Design review of the part built by this model. Coordinates are the model's own, in mm. Face numbers are marked on the shaded views. A direction names the side the tool comes from. Give positions to 0.01 mm unless a question says otherwise; leave off trailing zeros. Order: outer loops, then holes, each group sorted by start corner. A loop starts at its lowest first (then second) coordinate and runs counter-clockwise, first axis right, second up. Notation, with made-up numbers: (54, 74.5) -> (103, 74.5) arc R23 ccw to (103, 105.5) -> close; hole circle Ø9 at (-5, 12.25). An arc over 180 degrees is marked (long way). Return JSON: item names as keys, results as strings.
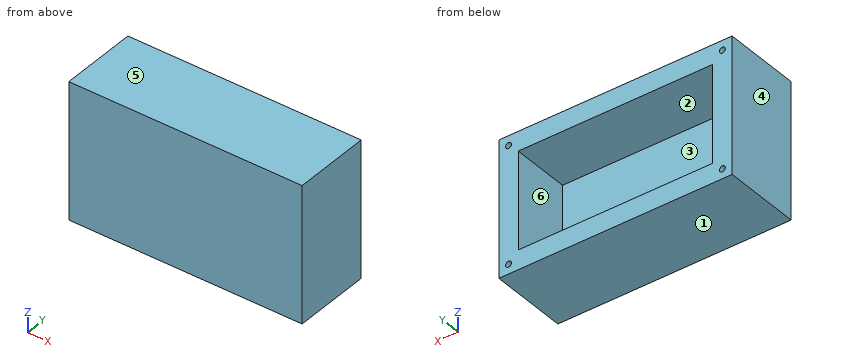
```python
from build123d import *

# Parameters (mm, degrees)
CROQUIS1_W              = 120
CROQUIS1_H              = 70
SALIENTE_EXTRUIR1_DEPTH = 40
CROQUIS2_W              = 100
CROQUIS2_H              = 50
CORTAR_EXTRUIR1_DEPTH   = 30
CROQUIS3_R              = 1.5
CORTAR_EXTRUIR2_DEPTH   = 10


with BuildPart() as part:
    # Croquis1 → Saliente-Extruir1 (new body)
    with BuildSketch(Plane(origin=(0, 0, 0), x_dir=(1, 0, 0), z_dir=(0, 1, 0))):
        Rectangle(CROQUIS1_W, CROQUIS1_H)
    extrude(amount=SALIENTE_EXTRUIR1_DEPTH)

    # Croquis2 → Cortar-Extruir1 (cut)
    with BuildSketch(Plane(origin=(0, 40, 0), x_dir=(1, 0, 0), z_dir=(0, 1, 0))):
        Rectangle(CROQUIS2_W, CROQUIS2_H)
    extrude(amount=-CORTAR_EXTRUIR1_DEPTH, mode=Mode.SUBTRACT)

    # Croquis3 → Cortar-Extruir2 (cut)
    with BuildSketch(Plane(origin=(0, 40, 0), x_dir=(1, 0, 0), z_dir=(0, 1, 0))):
        with Locations(Location((-55, -30, 0), (0, 0, 270))):
            Circle(CROQUIS3_R)
        with Locations(Location((-55, 30, 0), (0, 0, 270))):
            Circle(CROQUIS3_R)
        with Locations(Location((55, 30, 0), (0, 0, 270))):
            Circle(CROQUIS3_R)
        with Locations(Location((55, -30, 0), (0, 0, 270))):
            Circle(CROQUIS3_R)
    extrude(amount=-CORTAR_EXTRUIR2_DEPTH, mode=Mode.SUBTRACT)


solid = part.part
```
Item 1: Add section B-B (x = -55). Give the boundary of the cut face in (y, z).
Result set:
{"outline": "(0, -35) -> (40, -35) -> (40, -31.5) -> (30, -31.5) -> (30, -28.5) -> (40, -28.5) -> (40, 28.5) -> (30, 28.5) -> (30, 31.5) -> (40, 31.5) -> (40, 35) -> (0, 35) -> close"}
Item 2: Mouldability with a two-part tool opening along Z and no side actions: class the marked faces 3, 4, 5 and 6 as released by +Z, released by -Z, zero draft, split by the parting line, or undercut.
Result set:
{"face 3": "undercut", "face 4": "zero draft", "face 5": "released by +Z", "face 6": "undercut"}
Item 3: Add section A-A (y = 18). Give the boundary of the cut face in (x, z).
Result set:
{"outline": "(-60, -35) -> (60, -35) -> (60, 35) -> (-60, 35) -> close; hole (-50, -25) -> (50, -25) -> (50, 25) -> (-50, 25) -> close"}
Item 4: Wall thickness on L1, parallel to X at y = 33, z = -30; L2, parallel to Z at x = -11, y = 23; L3, parallel to X at y = 12, z = -19: over which ranges is each line inside the solid? List them lowest first. Write a range as [from, to].
Result set:
{"L1": "x = [-60, -56.5], [-53.5, 53.5], [56.5, 60]", "L2": "z = [-35, -25], [25, 35]", "L3": "x = [-60, -50], [50, 60]"}
Item 5: Add section D-D (x = 43). Give the boundary of the cut face in (y, z).
Result set:
{"outline": "(0, -35) -> (40, -35) -> (40, -25) -> (10, -25) -> (10, 25) -> (40, 25) -> (40, 35) -> (0, 35) -> close"}
Item 6: For pin 1 (1.8 mm diameter, centred on x = -55, z = 30, fed in from +Y); pin 2 (10 mm diameter, centred on x = 42.5, z = 0.5, fed in from +Y), all flat-tipped, find the tip position at first contact; note any pin that passes through.
Result set:
{"pin 1": "stops at y = 30", "pin 2": "stops at y = 10"}
Item 7: Add section C-C (z = 19.5). Give the boundary of the cut face in (x, y), plus the area to 3 significant figures.
Result set:
{"outline": "(-60, 0) -> (60, 0) -> (60, 40) -> (50, 40) -> (50, 10) -> (-50, 10) -> (-50, 40) -> (-60, 40) -> close", "area": "1,800 mm^2"}
Item 8: Machinability: for the marked faces 1 and 2, which of the approach directions +Z, -Z, +X, -X, +Y, -Y give a long, thin tool a straight path to every point of the face, cutting with its end or side? Answer none if there is none.
Result set:
{"face 1": "-Z, +X, -X, +Y, -Y", "face 2": "+Y"}
